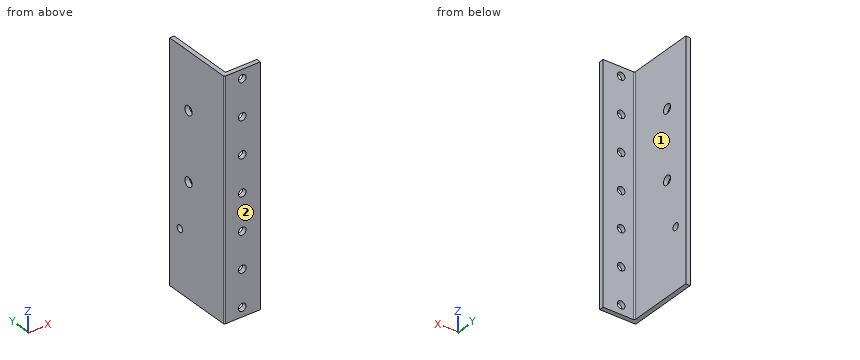
from build123d import *

# Parameters (mm, degrees)
BOSS_EXTRUDE1_DEPTH = 165.1
SKETCH3_R           = 2.667
CUT_EXTRUDE2_DEPTH  = 3.175
SKETCH4_R           = 3.302
CUT_EXTRUDE3_DEPTH  = 3.175
SKETCH5_R           = 2.4765
CUT_EXTRUDE4_DEPTH  = 6.35


with BuildPart() as part:
    # Sketch1 → Boss-Extrude1 (new body)
    with BuildSketch(Plane.XY):
        with BuildLine():
            Line((3.175, 50.8), (3.175, 3.937))
            ThreePointArc((3.175, 3.937), (3.398184633, 3.398184633), (3.937, 3.175))
            Line((3.937, 3.175), (25.4, 3.175))
            Line((25.4, 3.175), (25.4, 0))
            Line((25.4, 0), (0.762, 0))
            ThreePointArc((0.762, 0), (0.223184633, 0.223184633), (0, 0.762))
            Line((0, 0.762), (0, 50.8))
            Line((0, 50.8), (3.175, 50.8))
        make_face()
    extrude(amount=BOSS_EXTRUDE1_DEPTH)

    # Sketch3 → Cut-Extrude2 (cut)
    with BuildSketch(Plane.XZ):
        with Locations(Location((12.7, 6.42874, 0), (0, 0, 270))):
            Circle(SKETCH3_R)
        with Locations(Location((12.7, 31.82874, 0), (0, 0, 270))):
            Circle(SKETCH3_R)
        with Locations(Location((12.7, 57.22874, 0), (0, 0, 270))):
            Circle(SKETCH3_R)
        with Locations(Location((12.7, 82.62874, 0), (0, 0, 270))):
            Circle(SKETCH3_R)
        with Locations(Location((12.7, 108.02874, 0), (0, 0, 270))):
            Circle(SKETCH3_R)
        with Locations(Location((12.7, 133.42874, 0), (0, 0, 270))):
            Circle(SKETCH3_R)
        with Locations(Location((12.7, 158.82874, 0), (0, 0, 270))):
            Circle(SKETCH3_R)
    extrude(amount=-CUT_EXTRUDE2_DEPTH, mode=Mode.SUBTRACT)

    # Sketch4 → Cut-Extrude3 (cut)
    with BuildSketch(Plane(origin=(3.175, 0, 0), x_dir=(0, 0, -1), z_dir=(1, 0, 0))):
        with Locations(Location((-77.7875, 33.3375, 0), (0, 0, 90))):
            Circle(SKETCH4_R)
        with Locations(Location((-125.4125, 33.3375, 0), (0, 0, 90))):
            Circle(SKETCH4_R)
    extrude(amount=-CUT_EXTRUDE3_DEPTH, mode=Mode.SUBTRACT)

    # Sketch5 → Cut-Extrude4 (cut)
    with BuildSketch(Plane(origin=(6.35, 0, 0), x_dir=(0, 0, -1), z_dir=(1, 0, 0))):
        with Locations(Location((-42.773092, 41.347136, 0), (0, 0, 90))):
            Circle(SKETCH5_R)
    extrude(amount=-CUT_EXTRUDE4_DEPTH, mode=Mode.SUBTRACT)


solid = part.part
The listing builds one solid part. Answer for the finished solid, in the listing's coordinates (mm). Face numbers are marked on the shaded views. A direction names the side the tool comes from. Give positions to 0.01 mm unless a question says otherwise; leave off trailing zeros. Order: outer loops, then holes, each group sorted by start corner. A loop starts at its lowest first (then second) coordinate and runs counter-clockwise, first axis right, second up. Notation, with made-up numbers: (60, 51.5) -> (118, 51.5) arc R9 cw to (118, 56.5) -> close; hole circle Ø3 at (49.5, 81.5). An arc over 180 degrees is marked (long way). Put each result on its own line as item: value.
Item 1: Straight lines are drawn through the part: line 1 (X direction, y = 11, z = 137) (3 decimals); line 2 (Y direction, x = 3.5, z = 84). For each, find the intervals that lie inside material, in ascending order.
Established:
line 1: x = 0 to 3.175
line 2: y = 0 to 3.31
Item 2: For the marked faces 1 and 2, determine the directions among +Z, -Z, +X, -X, +Y, -Y from which every point of the face is accessible in a straight line to the end or side of a thin tool.
Established:
face 1: +Z, -Z, +X, +Y
face 2: +Z, -Z, +X, -X, -Y
Item 3: A cutting plane is placed at B-B on z = 48. Give the vertices of the cut face in (x, y) (3 decimals), plus the area to 3 significant figures.
Established:
outline: (0, 0.762) arc R0.762 ccw to (0.762, 0) -> (25.4, 0) -> (25.4, 3.175) -> (3.937, 3.175) arc R0.762 cw to (3.175, 3.937) -> (3.175, 50.8) -> (0, 50.8) -> close
area: 232 mm^2
Item 4: A cutting plane is placed at C-C on x = 23. Give the vertices of the cut face in (y, z) (3 decimals).
Established:
outline: (0, 0) -> (3.175, 0) -> (3.175, 165.1) -> (0, 165.1) -> close
Item 5: A cutting plane is placed at A-A on x = 12.7. Count the separate pieces of the cut face and the enclosed holes in it, plus the area to 3 significant figures.
Established:
separate pieces: 8
enclosed holes: 0
area: 406 mm^2
Item 6: Given P1, Ø6, axis at x = 12.7, z = 133.43, coming from the +Y side (3 decimals); P2, Ø4.5, axis at x = 12.7, z = 82.63, coming from the -Y side; P3, Ø12, axis at y = 10.5, z = 128, coming from the +X side (3 decimals), each flat-ended and moving along its own axis, determine where each tip first touches the part or whether it passes through.
Established:
P1: stops at y = 3.175
P2: passes through
P3: stops at x = 3.175
